from build123d import *

# Parameters (mm, degrees)
SKETCH1_R                  = 1.5
BOSS_EXTRUDE1_DEPTH        = 2.5
SKETCH1_3_R                = 1
CUT_EXTRUDE1_DEPTH         = 2
BOSS_EXTRUDE2_DEPTH        = 0.375
BOSS_EXTRUDE2_DEPTH_BACK   = 0.375
BOSS_EXTRUDE2_2_DEPTH      = 0.375
BOSS_EXTRUDE2_2_DEPTH_BACK = 0.375
BOSS_EXTRUDE3_START        = -0.381966
SKETCH2_W                  = 0.75
SKETCH2_H                  = 2
BOSS_EXTRUDE3_DEPTH        = 0.381966
SKETCH4_W                  = 0.75
SKETCH4_H                  = 2
BOSS_EXTRUDE4_DEPTH        = 0.381966
CUT_EXTRUDE2_REACH         = 3.625
SKETCH5_R                  = 0.25
SKETCH5_R_2                = 0.3
SKETCH5_R_3                = 0.35
SKETCH5_R_4                = 0.4
SKETCH5_R_5                = 0.45
SKETCH5_R_6                = 0.5


with BuildPart() as part:
    # Sketch1 → Boss-Extrude1 (new body)
    with BuildSketch(Plane.XY):
        Circle(SKETCH1_R)
    extrude(amount=BOSS_EXTRUDE1_DEPTH)

    # Sketch1<3> → Cut-Extrude1 (cut)
    with BuildSketch(Plane.XY):
        Circle(SKETCH1_3_R)
    extrude(amount=CUT_EXTRUDE1_DEPTH, mode=Mode.SUBTRACT)



with BuildPart() as body_2:
    # Sketch3 → Boss-Extrude2 (new body, two sides)
    with BuildSketch(Plane(origin=(0, 0, 1.25), x_dir=(0, -1, 0), z_dir=(0, 0, -1))) as boss_extrude2_sk:
        with BuildLine():
            Line((1, 1.5), (0.75, 11.5))
            ThreePointArc((0.75, 11.5), (0, 12.25), (-0.75, 11.5))
            Line((-0.75, 11.5), (-1, 1.5))
            Line((-1, 1.5), (1, 1.5))
        make_face()
    extrude(amount=BOSS_EXTRUDE2_DEPTH)
    extrude(boss_extrude2_sk.sketch, amount=-BOSS_EXTRUDE2_DEPTH_BACK)


with BuildPart() as body_3:
    # Sketch3 → Boss-Extrude2 2 (new body, two sides)
    with BuildSketch(Plane(origin=(0, 0, 1.25), x_dir=(0, -1, 0), z_dir=(0, 0, -1))) as boss_extrude2_2_sk:
        with BuildLine():
            Line((-1, -1.5), (-0.75, -11.5))
            ThreePointArc((-0.75, -11.5), (0, -12.25), (0.75, -11.5))
            Line((0.75, -11.5), (1, -1.5))
            Line((1, -1.5), (-1, -1.5))
        make_face()
    extrude(amount=BOSS_EXTRUDE2_2_DEPTH)
    extrude(boss_extrude2_2_sk.sketch, amount=-BOSS_EXTRUDE2_2_DEPTH_BACK)


with BuildPart() as part_1:
    add(part.part)

    add(body_2.part)  # Boss-Extrude3 merges body 2
    # Sketch2 → Boss-Extrude3 (add)
    with BuildSketch(Plane.ZY.offset(1.5).offset(BOSS_EXTRUDE3_START)):
        with Locations((1.25, 0)):
            Rectangle(SKETCH2_W, SKETCH2_H)
    extrude(amount=BOSS_EXTRUDE3_DEPTH)


    add(body_3.part)  # Boss-Extrude4 merges body 3
    # Sketch4 → Boss-Extrude4 (add)
    with BuildSketch(Plane.ZY.offset(-1.5)):
        with Locations((1.25, 0)):
            Rectangle(SKETCH4_W, SKETCH4_H)
    extrude(amount=BOSS_EXTRUDE4_DEPTH)

    # Sketch5 → Cut-Extrude2 (cut, up to next)
    with BuildSketch(Plane.XY.offset(1.625), mode=Mode.PRIVATE) as cut_extrude2_sk1:
        with Locations((-10.8, 0)):
            Circle(SKETCH5_R)
    cut_extrude2_tool1 = extrude(cut_extrude2_sk1.sketch, amount=-CUT_EXTRUDE2_REACH, mode=Mode.PRIVATE) & part_1.part
    add(cut_extrude2_tool1.solids().sort_by_distance((-10.8, 0, 1.625))[0], mode=Mode.SUBTRACT)
    # Sketch5 → Cut-Extrude2 (cut, up to next)
    with BuildSketch(Plane.XY.offset(1.625), mode=Mode.PRIVATE) as cut_extrude2_sk2:
        with Locations((-9.5, 0)):
            Circle(SKETCH5_R_2)
    cut_extrude2_tool2 = extrude(cut_extrude2_sk2.sketch, amount=-CUT_EXTRUDE2_REACH, mode=Mode.PRIVATE) & part_1.part
    add(cut_extrude2_tool2.solids().sort_by_distance((-9.5, 0, 1.625))[0], mode=Mode.SUBTRACT)
    # Sketch5 → Cut-Extrude2 (cut, up to next)
    with BuildSketch(Plane.XY.offset(1.625), mode=Mode.PRIVATE) as cut_extrude2_sk3:
        with Locations((-8, 0)):
            Circle(SKETCH5_R_3)
    cut_extrude2_tool3 = extrude(cut_extrude2_sk3.sketch, amount=-CUT_EXTRUDE2_REACH, mode=Mode.PRIVATE) & part_1.part
    add(cut_extrude2_tool3.solids().sort_by_distance((-8, 0, 1.625))[0], mode=Mode.SUBTRACT)
    # Sketch5 → Cut-Extrude2 (cut, up to next)
    with BuildSketch(Plane.XY.offset(1.625), mode=Mode.PRIVATE) as cut_extrude2_sk4:
        with Locations((-6.5, 0)):
            Circle(SKETCH5_R_4)
    cut_extrude2_tool4 = extrude(cut_extrude2_sk4.sketch, amount=-CUT_EXTRUDE2_REACH, mode=Mode.PRIVATE) & part_1.part
    add(cut_extrude2_tool4.solids().sort_by_distance((-6.5, 0, 1.625))[0], mode=Mode.SUBTRACT)
    # Sketch5 → Cut-Extrude2 (cut, up to next)
    with BuildSketch(Plane.XY.offset(1.625), mode=Mode.PRIVATE) as cut_extrude2_sk5:
        with Locations((-4.75, 0)):
            Circle(SKETCH5_R_5)
    cut_extrude2_tool5 = extrude(cut_extrude2_sk5.sketch, amount=-CUT_EXTRUDE2_REACH, mode=Mode.PRIVATE) & part_1.part
    add(cut_extrude2_tool5.solids().sort_by_distance((-4.75, 0, 1.625))[0], mode=Mode.SUBTRACT)
    # Sketch5 → Cut-Extrude2 (cut, up to next)
    with BuildSketch(Plane.XY.offset(1.625), mode=Mode.PRIVATE) as cut_extrude2_sk6:
        with Locations((-3, 0)):
            Circle(SKETCH5_R_6)
    cut_extrude2_tool6 = extrude(cut_extrude2_sk6.sketch, amount=-CUT_EXTRUDE2_REACH, mode=Mode.PRIVATE) & part_1.part
    add(cut_extrude2_tool6.solids().sort_by_distance((-3, 0, 1.625))[0], mode=Mode.SUBTRACT)
    # Sketch5 → Cut-Extrude2 (cut, up to next)
    with BuildSketch(Plane.XY.offset(1.625), mode=Mode.PRIVATE) as cut_extrude2_sk7:
        with Locations((3, 0)):
            Circle(SKETCH5_R_6)
    cut_extrude2_tool7 = extrude(cut_extrude2_sk7.sketch, amount=-CUT_EXTRUDE2_REACH, mode=Mode.PRIVATE) & part_1.part
    add(cut_extrude2_tool7.solids().sort_by_distance((3, 0, 1.625))[0], mode=Mode.SUBTRACT)
    # Sketch5 → Cut-Extrude2 (cut, up to next)
    with BuildSketch(Plane.XY.offset(1.625), mode=Mode.PRIVATE) as cut_extrude2_sk8:
        with Locations((4.75, 0)):
            Circle(SKETCH5_R_5)
    cut_extrude2_tool8 = extrude(cut_extrude2_sk8.sketch, amount=-CUT_EXTRUDE2_REACH, mode=Mode.PRIVATE) & part_1.part
    add(cut_extrude2_tool8.solids().sort_by_distance((4.75, 0, 1.625))[0], mode=Mode.SUBTRACT)
    # Sketch5 → Cut-Extrude2 (cut, up to next)
    with BuildSketch(Plane.XY.offset(1.625), mode=Mode.PRIVATE) as cut_extrude2_sk9:
        with Locations((6.5, 0)):
            Circle(SKETCH5_R_4)
    cut_extrude2_tool9 = extrude(cut_extrude2_sk9.sketch, amount=-CUT_EXTRUDE2_REACH, mode=Mode.PRIVATE) & part_1.part
    add(cut_extrude2_tool9.solids().sort_by_distance((6.5, 0, 1.625))[0], mode=Mode.SUBTRACT)
    # Sketch5 → Cut-Extrude2 (cut, up to next)
    with BuildSketch(Plane.XY.offset(1.625), mode=Mode.PRIVATE) as cut_extrude2_sk10:
        with Locations((8, 0)):
            Circle(SKETCH5_R_3)
    cut_extrude2_tool10 = extrude(cut_extrude2_sk10.sketch, amount=-CUT_EXTRUDE2_REACH, mode=Mode.PRIVATE) & part_1.part
    add(cut_extrude2_tool10.solids().sort_by_distance((8, 0, 1.625))[0], mode=Mode.SUBTRACT)
    # Sketch5 → Cut-Extrude2 (cut, up to next)
    with BuildSketch(Plane.XY.offset(1.625), mode=Mode.PRIVATE) as cut_extrude2_sk11:
        with Locations((9.5, 0)):
            Circle(SKETCH5_R_2)
    cut_extrude2_tool11 = extrude(cut_extrude2_sk11.sketch, amount=-CUT_EXTRUDE2_REACH, mode=Mode.PRIVATE) & part_1.part
    add(cut_extrude2_tool11.solids().sort_by_distance((9.5, 0, 1.625))[0], mode=Mode.SUBTRACT)
    # Sketch5 → Cut-Extrude2 (cut, up to next)
    with BuildSketch(Plane.XY.offset(1.625), mode=Mode.PRIVATE) as cut_extrude2_sk12:
        with Locations((10.8, 0)):
            Circle(SKETCH5_R)
    cut_extrude2_tool12 = extrude(cut_extrude2_sk12.sketch, amount=-CUT_EXTRUDE2_REACH, mode=Mode.PRIVATE) & part_1.part
    add(cut_extrude2_tool12.solids().sort_by_distance((10.8, 0, 1.625))[0], mode=Mode.SUBTRACT)


solid = part_1.part
The listing builds one solid part. Answer for the finished solid, in the listing's coordinates (mm). A direction names the side the tool comes from. Round coordinates to 2 decimals unless told otherwise and drop trailing zeros. Order: outer loops, then holes, each group sorted by start corner. A loop starts at its lowest first (then second) coordinate and runs counter-clockwise, first axis right, second up. Notation, with made-up numbers: M 65.5,64 L 72.5,64 A37 cw 72.5,100 Z; hole C 7.25,-29.75 d1. An arc over 180 degrees is marked long. Answer in a Markdown table with one row per item. Add a question column.
1) Flat-ended cylindrical pins translate along their axes: pin 1 Ø1.6 at (x, y) = (0, 0) entering from -Z; pin 2 Ø1 at (x, y) = (8.5, 0) entering from +Z (3 decimals); pin 3 Ø0.6 at (x, y) = (-4.5, -0.5) entering from -Z (3 decimals). Find the tip coordinate at first contact, or state that the pin passes through.
2) The part is cut by section B-B on z = 0.25. Determine the outline of the cut face in (x, y), plus the area to 3 significant figures.
3) Consider line 1 along X through (y, z) = (-0.05, 0.45); line 2 along Z through (x, y) = (-1.5, -0.85) (3 decimals); line 3 along Y through (x, z) = (-1.5, 0.95). Determine where each line is inside the solid, lowest interval first. Write a range as from..to.
4) The part is cut by section C-C on x = 0. Determine the outline of the cut face in (y, z), plus the area to 3 significant figures.
5) The part is cut by section D-D on y = 0. Count the separate pieces of the cut face and the enclosed holes in it, plus the area to 3 significant figures.
6) Which of the six approach directions +Z, -Z, +X, -X, +Y, -Y give full straight-line access (tool end or side, diameter ignored) to faces 1 (the face through (0, 0, 2.5)), 2 (the face through (0, 0, 2))?
7) Determine the mould class of faces 3 (the face through (-0.195, 1.487, 1.232)), 4 (the face through (0, -1, 1)), 5 (the face through (6.8, -0.5, 0.875)) for opening direction Y: pulls with the +Y half, pulls with the -Y half, needs draft (parallel to the pull), parting line crosses it, or undercut.
8) The part is cut by section A-A on x = 9.5. Determine the outline of the cut face in (y, z) (3 decimals), plus the area to 3 significant figures.
Findings below:
| question | item | result |
|---|---|---|
| 1 | pin 1 | stops at z = 2 |
| 1 | pin 2 | stops at z = 1.625 |
| 1 | pin 3 | stops at z = 0.875 |
| 2 | outline | C 0,0 d3; hole C 0,0 d2 |
| 2 | area | 3.93 mm² |
| 3 | line 1 | x = -1.5..-1, 1..1.5 |
| 3 | line 2 | z = 0.875..1.625 |
| 3 | line 3 | y = -1..1 |
| 4 | outline | M -1.5,0 L -1,0 L -1,2 L 1,2 L 1,0 L 1.5,0 L 1.5,2.5 L -1.5,2.5 Z |
| 4 | area | 3.50 mm² |
| 5 | separate pieces | 13 |
| 5 | enclosed holes | 0 |
| 5 | area | 12.9 mm² |
| 6 | face 1 | +Z, +X, -X, +Y, -Y |
| 6 | face 2 | -Z |
| 7 | face 3 | parting line crosses it |
| 7 | face 4 | undercut |
| 7 | face 5 | needs draft |
| 8 | outline | M -0.8,0.875 L -0.3,0.875 L -0.3,1.625 L -0.8,1.625 Z; M 0.3,0.875 L 0.8,0.875 L 0.8,1.625 L 0.3,1.625 Z |
| 8 | area | 0.750 mm² |
